Verification items for the finished model (mm, model axes). A direction names the side the tool comes from. Give positions to 0.01 mm unless a question says otherwise; leave off trailing zeros. Loops run counter-clockwise (first coordinate to the right, second up) from the corner with the lowest first, then second, coordinate; pieces in that order, holes last. Notation, with made-up numbers: M -25,68 L -16,68 A10 cw -16,79 Z; hole C -3,-31 d7. An arc over 180 degrees is marked long. Use a Markdown table: item, result.
from build123d import *

# Parameters (mm, degrees)
BOSS_EXTRUDE1_DEPTH = 5
BOSS_EXTRUDE2_REACH = 104.182
SKETCH3_R           = 15
SKETCH3_R_2         = 12.5
BOSS_EXTRUDE3_REACH = 104.182
SKETCH4_R           = 1
CIRPATTERN1_START   = 1.089571064
CIRPATTERN1_DEPTH   = 61.685010975
CIRPATTERN1_START_2 = -13.151834357
CIRPATTERN1_2_DEPTH = 16.804980917
CIRPATTERN1_START_3 = -6.049458183
CIRPATTERN1_3_DEPTH = 9.702604743
RIB2_REACH          = 89.235
SKETCH5_WALL_W      = 196.470282612
SKETCH5_WALL_H      = 3
RIB3_REACH          = 101.962
SKETCH6_WALL_W      = 240.643320444
SKETCH6_WALL_H      = 3
SKETCH7_R           = 1.5
CUT_EXTRUDE1_DEPTH  = 5


with BuildPart() as part:
    # Sketch2 → Boss-Extrude1 (new body)
    with BuildSketch(Plane(origin=(0, 0, 0), x_dir=(1, 0, 0), z_dir=(0, 1, 0))):
        with BuildLine():
            Line((35, 20), (-35, 20))
            ThreePointArc((-35, 20), (-45.606601718, 15.606601718), (-50, 5))
            Line((-50, 5), (-50, -5))
            ThreePointArc((-50, -5), (-45.606601718, -15.606601718), (-35, -20))
            Line((-35, -20), (35, -20))
            ThreePointArc((35, -20), (45.606601718, -15.606601718), (50, -5))
            Line((50, -5), (50, 5))
            ThreePointArc((50, 5), (45.606601718, 15.606601718), (35, 20))
        make_face()
    extrude(amount=BOSS_EXTRUDE1_DEPTH)

    # Boss-Extrude2: up to this plane
    boss_extrude2_end = Plane(origin=(35, 5, 5), z_dir=(0, -1, 0))
    # Sketch3 → Boss-Extrude2 (add, up to the surface)
    with BuildSketch(Plane(origin=(36.006021059, 51.421927207, 0), x_dir=(0, 0, -1), z_dir=(0.5735764363510473, 0.819152044288991, 0)), mode=Mode.PRIVATE) as boss_extrude2_sk1:
        with Locations(Location((0, 15, 0), (0, 0, 90))):
            Circle(SKETCH3_R)
        with Locations(Location((0, 15, 0), (0, 0, 90))):
            Circle(SKETCH3_R_2, mode=Mode.SUBTRACT)
    boss_extrude2_tool1 = split(extrude(boss_extrude2_sk1.sketch, amount=-BOSS_EXTRUDE2_REACH, mode=Mode.PRIVATE), bisect_by=boss_extrude2_end, keep=Keep.BOTH, mode=Mode.PRIVATE)
    add(boss_extrude2_tool1.solids().sort_by_distance((35.658484, 51.665275, 0))[0])

    # Boss-Extrude3: up to this plane
    boss_extrude3_end = Plane(origin=(35, 5, 5), z_dir=(0, -1, 0))
    # Sketch4 → Boss-Extrude3 (add, up to the surface)
    with BuildSketch(Plane(origin=(36.006021059, 51.421927207, 0), x_dir=(0.819152044288991, -0.5735764363510474, 0), z_dir=(0.5735764363510474, 0.819152044288991, 0)), mode=Mode.PRIVATE) as boss_extrude3_sk1:
        with Locations((-15, 12.5)):
            Circle(SKETCH4_R)
    boss_extrude3_tool1 = split(extrude(boss_extrude3_sk1.sketch, amount=-BOSS_EXTRUDE3_REACH, mode=Mode.PRIVATE), bisect_by=boss_extrude3_end, keep=Keep.BOTH, mode=Mode.PRIVATE)
    add(boss_extrude3_tool1.solids().sort_by_distance((23.71874, 60.025574, -12.5))[0])

    # CirPattern1: read off the stored shape, not the designer's step
    # CirPattern1 outline → CirPattern1 (add)
    with BuildSketch(Plane(origin=(0, 0, 0), x_dir=(0.819152044288991, -0.5735764363510472, 0), z_dir=(0.5735764363510472, 0.8191520442889911, 0)).offset(CIRPATTERN1_START)):
        with BuildLine():
            ThreePointArc((-5.482908637, 8.104009624), (-6.161165235, 8.838834765), (-6.895990376, 9.517091363))
            ThreePointArc((-6.895990376, 9.517091363), (-6.868272016, 8.131727984), (-5.482908637, 8.104009624))
        make_face()
        with BuildLine():
            ThreePointArc((-23.104009624, 9.517091363), (-23.838834765, 8.838834765), (-24.517091363, 8.104009624))
            ThreePointArc((-24.517091363, 8.104009624), (-23.131727984, 8.131727984), (-23.104009624, 9.517091363))
        make_face()
        with BuildLine():
            ThreePointArc((-27.46, 0.99919968), (-27.5, 0), (-27.46, -0.99919968))
            ThreePointArc((-27.46, -0.99919968), (-26.5, 0), (-27.46, 0.99919968))
        make_face()
        with BuildLine():
            ThreePointArc((-24.517091363, -8.104009624), (-23.838834765, -8.838834765), (-23.104009624, -9.517091363))
            ThreePointArc((-23.104009624, -9.517091363), (-23.131727984, -8.131727984), (-24.517091363, -8.104009624))
        make_face()
        with BuildLine():
            ThreePointArc((-15.99919968, -12.46), (-15, -12.5), (-14.00080032, -12.46))
            ThreePointArc((-14.00080032, -12.46), (-15, -11.5), (-15.99919968, -12.46))
        make_face()
        with BuildLine():
            ThreePointArc((-6.895990376, -9.517091363), (-6.161165235, -8.838834765), (-5.482908637, -8.104009624))
            ThreePointArc((-5.482908637, -8.104009624), (-6.868272016, -8.131727984), (-6.895990376, -9.517091363))
        make_face()
        with BuildLine():
            ThreePointArc((-2.54, -0.99919968), (-2.5, 0), (-2.54, 0.99919968))
            ThreePointArc((-2.54, 0.99919968), (-3.5, 0), (-2.54, -0.99919968))
        make_face()
    extrude(amount=CIRPATTERN1_DEPTH)

    # CirPattern1 2 outline → CirPattern1 2 (add)
    with BuildSketch(Plane(origin=(0, 0, 0), x_dir=(0.819152044288991, -0.5735764363510472, 0), z_dir=(0.5735764363510472, 0.8191520442889911, 0)).offset(CIRPATTERN1_START_2)):
        with BuildLine():
            ThreePointArc((-23.104009624, 9.517091363), (-23.838834765, 8.838834765), (-24.517091363, 8.104009624))
            ThreePointArc((-24.517091363, 8.104009624), (-23.131727984, 8.131727984), (-23.104009624, 9.517091363))
        make_face()
        with BuildLine():
            ThreePointArc((-27.46, 0.99919968), (-27.5, 0), (-27.46, -0.99919968))
            ThreePointArc((-27.46, -0.99919968), (-26.5, 0), (-27.46, 0.99919968))
        make_face()
        with BuildLine():
            ThreePointArc((-24.517091363, -8.104009624), (-23.838834765, -8.838834765), (-23.104009624, -9.517091363))
            ThreePointArc((-23.104009624, -9.517091363), (-23.131727984, -8.131727984), (-24.517091363, -8.104009624))
        make_face()
    extrude(amount=CIRPATTERN1_2_DEPTH)

    # CirPattern1 3 outline → CirPattern1 3 (add)
    with BuildSketch(Plane(origin=(0, 0, 0), x_dir=(0.819152044288991, -0.5735764363510472, 0), z_dir=(0.5735764363510472, 0.8191520442889911, 0)).offset(CIRPATTERN1_START_3)):
        with BuildLine():
            ThreePointArc((-15.99919968, -12.46), (-15, -12.5), (-14.00080032, -12.46))
            ThreePointArc((-14.00080032, -12.46), (-15, -11.5), (-15.99919968, -12.46))
        make_face()
    extrude(amount=CIRPATTERN1_3_DEPTH)

    # Sketch5 wall → Rib2 (add, up to next)
    with BuildSketch(Plane(origin=(32.411809549, 19.659258263, 0), x_dir=(0.258819045097, -0.96592582629, 0), z_dir=(0.96592582629, 0.258819045097, 0)), mode=Mode.PRIVATE) as rib2_sk1:
        Rectangle(SKETCH5_WALL_W, SKETCH5_WALL_H)
    rib2_tool1 = extrude(rib2_sk1.sketch, amount=-RIB2_REACH, mode=Mode.PRIVATE) - part.part
    add(rib2_tool1.solids().sort_by_distance((32.411809549, 19.659258263, 0))[0])

    # Sketch6 wall → Rib3 (add, up to next)
    with BuildSketch(Plane(origin=(19.874497756, 22.00680033, 10.75), x_dir=(0, -0.878468996126, 0.47779935417), z_dir=(0, -0.47779935417, -0.878468996126)), mode=Mode.PRIVATE) as rib3_sk1:
        Rectangle(SKETCH6_WALL_W, SKETCH6_WALL_H)
    rib3_tool1 = extrude(rib3_sk1.sketch, amount=RIB3_REACH, mode=Mode.PRIVATE) - part.part
    rib3 = rib3_tool1.solids().sort_by_distance((19.874497756, 22.00680033, 10.75))[0]
    add(rib3)

    # Mirror1: Rib3 across plane
    add(rib3.mirror(Plane.XY))

    # Sketch7 → Cut-Extrude1 (cut)
    with BuildSketch(Plane.XZ):
        with Locations(Location((-40, 0, 0), (0, 0, 270))):
            Circle(SKETCH7_R)
        with Locations(Location((40, -12.5, 0), (0, 0, 270))):
            Circle(SKETCH7_R)
        with Locations(Location((40, 12.5, 0), (0, 0, 270))):
            Circle(SKETCH7_R)
    extrude(amount=-CUT_EXTRUDE1_DEPTH, mode=Mode.SUBTRACT)


solid = part.part
(1) Set-up check for faces 5 (the flat face through (-15, 5, 0)), 6 (the flat face through (19.85, 18.77, -12.51)), 7 (the flat face through (18.374, 14, 8)), 8 (the flat face through (31.72, 22.24, -0.02)): record each of +Z, -Z, +X, -X, +Y, -Y from which the full face is reachable in a straight line by a thin tool's end or side.
Results below:
| item | result |
|---|---|
| face 5 | none |
| face 6 | -Z, +X |
| face 7 | +Z |
| face 8 | +Z, -Z, +X |
(2) Cross-section at B-B on x = 40. Record the cut outline in (y, z), then the cut area to 3 significant figures.
Results below:
| item | result |
|---|---|
| outline | M 0,-19.14 L 5,-19.14 L 5,-14 L 0,-14 Z; M 0,-11 L 5,-11 L 5,11 L 0,11 Z; M 0,14 L 5,14 L 5,19.14 L 0,19.14 Z |
| area | 161 mm^2 |
(3) Gauge pin test, flat ends, axial feed: P1, Ø1, axis at x = 16.5, y = 53.5, coming from the -Z side; P2, Ø5, axis at x = -11, z = -7, coming from the -Y side; P3, Ø4.5, axis at x = 9, y = 20, coming from the -Z side; P4, Ø3, axis at x = 0, y = 29.5, coming from the +Z side. Record the tip position at first contact, or that the pin passes through.
Results below:
| item | result |
|---|---|
| P1 | z = -14.91 |
| P2 | y = 0 |
| P3 | z = -12.25 |
| P4 | z = 14.99 |
(4) Cross-section at A-A on x = -40. Record the cut outline in (y, z), then the cut area to 3 significant figures.
Results below:
| item | result |
|---|---|
| outline | M 0,-19.14 L 5,-19.14 L 5,-1.5 L 0,-1.5 Z; M 0,1.5 L 5,1.5 L 5,19.14 L 0,19.14 Z |
| area | 176 mm^2 |
(5) Material ranges on line 1 (X direction, y = 2.5, z = 0); line 2 (X direction, y = 2.4, z = 12.5); line 3 (X direction, y = 23, z = 7), recorded low to high.
Results below:
| item | result |
|---|---|
| line 1 | -50 to -41.5, -38.5 to 50 |
| line 2 | -47.99 to 38.5, 41.5 to 47.99 |
| line 3 | -18.4 to -14.85, 10.44 to 13.99, 18.37 to 21.37 |
(6) Cross-section at C-C on z = 3. Record the cut outline in (x, y).
Results below:
| item | result |
|---|---|
| outline | M -50,0 L 50,0 L 50,5 L 21.37,5 L 21.37,31.05 L 35.76,51.6 L 33.66,53.07 L 0,5 L -29.62,5 L 13.78,66.99 L 11.68,68.46 L -32.75,5 L -50,5 Z; hole M 3.13,5 L 18.37,5 L 18.37,26.77 Z |
(7) Cross-section at D-D on z = 17. Record the cut outline in (x, y).
Results below:
| item | result |
|---|---|
| outline | M -44,0 L 44,0 L 44,5 L 21.37,5 L 21.37,10.52 L 18.37,10.52 L 18.37,5 L -44,5 Z |
(8) Draft check along X on faces 1 (the flat face through (-24, 5, -14)), 2 (the flat face through (21.374, 16, -7)), 3 (the cylindrical face through (15.908, 28.82, -0.021)), 4 (the flat face through (0, 2, 20)). Enter one of: +X half, -X half, draft (parallel to the pull), parting line (faces both ways), or undercut.
Results below:
| item | result |
|---|---|
| face 1 | undercut |
| face 2 | +X half |
| face 3 | undercut |
| face 4 | draft |
